The model under review builds one solid part; all positions refer to its coordinate system, in mm. Face numbers are marked on the shaded views. A direction names the side the tool comes from. Coordinates: 2 decimals unless noted, no trailing zeros. Loops run counter-clockwise (first coordinate to the right, second up) from the corner with the lowest first, then second, coordinate; pieces in that order, holes last. Notation, with made-up numbers: M -15.75,0 L 25.25,0 A24 ccw 25.25,14 Z; hole C 59,-26.75 d8. An arc over 180 degrees is marked long. Use one line per item in the form item = value.
```python
from build123d import *

# Parameters (mm, degrees)
SKETCH1_W           = 83
SKETCH1_H           = 59
BOSS_EXTRUDE1_DEPTH = 3
SKETCH2_W           = 83
SKETCH2_H           = 59
BOSS_EXTRUDE2_DEPTH = 23


with BuildPart() as part:
    # Sketch1 → Boss-Extrude1 (new body)
    with BuildSketch(Plane(origin=(0, 0, 0), x_dir=(1, 0, 0), z_dir=(0, 1, 0))):
        with Locations((41.5, 29.5)):
            Rectangle(SKETCH1_W, SKETCH1_H)
    extrude(amount=BOSS_EXTRUDE1_DEPTH)

    # Sketch2 → Boss-Extrude2 (add)
    with BuildSketch(Plane(origin=(0, 3, 0), x_dir=(1, 0, 0), z_dir=(0, 1, 0))):
        with Locations((41.5, 29.5)):
            Rectangle(SKETCH2_W, SKETCH2_H)
        with BuildLine():
            Line((3, 46.5), (3, 12.5))
            ThreePointArc((3, 12.5), (9.717514421, 9.717514421), (12.5, 3))
            Line((12.5, 3), (70.5, 3))
            ThreePointArc((70.5, 3), (73.282485579, 9.717514421), (80, 12.5))
            Line((80, 12.5), (80, 46.5))
            ThreePointArc((80, 46.5), (73.282485579, 49.282485579), (70.5, 56))
            Line((70.5, 56), (12.5, 56))
            ThreePointArc((12.5, 56), (9.717514421, 49.282485579), (3, 46.5))
        make_face(mode=Mode.SUBTRACT)
    extrude(amount=BOSS_EXTRUDE2_DEPTH)


solid = part.part
```
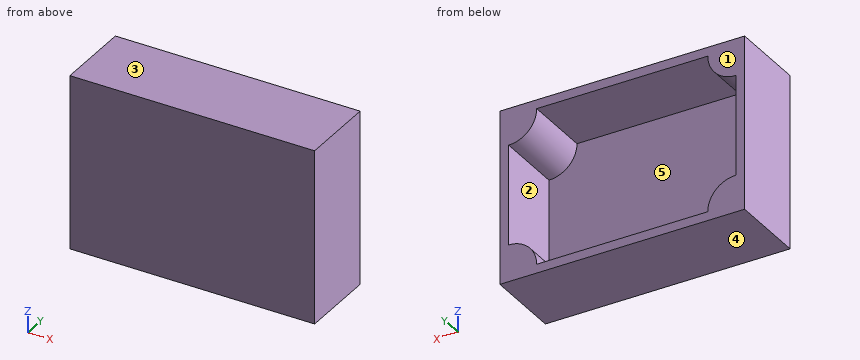
1. Add section C-C (x = 31). State the section outline as (y, z) points.
Response values:
outline = M 0,-59 L 26,-59 L 26,-56 L 3,-56 L 3,-3 L 26,-3 L 26,0 L 0,0 Z
2. Machinability: for the marked faces 1 and 2, which of the approach directions +Z, -Z, +X, -X, +Y, -Y give a long, thin tool a straight path to every point of the face, cutting with its end or side? Answer none if there is none.
Response values:
face_1 = +Z, -Z, +X, -X, +Y
face_2 = +Y
3. Wall thickness on line 1 along X through (y, z) = (18, -42); line 2 along Z through (x, y) = (62.5, 6); line 3 along Y through (x, z) = (53.5, -19.5): over which ranges is each line inside the solid? List them lowest first. Write a range as from..to.
Response values:
line_1 = 0..3, 80..83
line_2 = -59..-56, -3..0
line_3 = 0..3
4. Add section B-B (z = -45.5). State the section outline as (x, y) points.
Response values:
outline = M 0,0 L 83,0 L 83,26 L 80,26 L 80,3 L 3,3 L 3,26 L 0,26 Z
5. The part is to be moulded in two halves that separate along Z. For the marked faces 3, 4 and 5, say which applies: pulls with the +Z half, pulls with the -Z half, needs draft (parallel to the pull), parting line crosses it, or undercut.
Response values:
face_3 = pulls with the +Z half
face_4 = pulls with the -Z half
face_5 = undercut
6. Add section A-A (y = 17.5). State the section outline as (x, z) points, then the cut area to 3 significant figures.
Response values:
outline = M 0,-59 L 83,-59 L 83,0 L 0,0 Z; hole M 3,-46.5 A9.5 cw 12.5,-56 L 70.5,-56 A9.5 cw 80,-46.5 L 80,-12.5 A9.5 cw 70.5,-3 L 12.5,-3 A9.5 cw 3,-12.5 Z
area = 1,100 mm^2
7. Insertion check: P1, Ø11.5, axis at x = 51, y = 16, coming from the +Z side; P2, Ø16, axis at x = 31.5, z = -38, coming from the +Y side. Each pin has a flat end and moves straight along its axis. Give the tip position at first contact, or say it passes through.
Response values:
P1 = 0
P2 = 3
